Autodesk Inventor part; units mm, degrees
ref_plane "YZ Plane" through (0, 0, 0) normal (1, 0, 0) x (0, 1, 0)
ref_plane "XZ Plane" through (0, 0, 0) normal (0, 1, 0) x (-1, 0, 0)
ref_plane "XY Plane" through (0, 0, 0) normal (0, 0, 1) x (1, 0, 0)
sketch "Sketch1" plane through (0, 0, 0) normal (0, 1, 0) x (-1, 0, 0)
  line L0 (0, 0) -> (6, 0)
  line L1 (6, 0) -> (6, -3.7)
  line L2 (6, -3.7) -> (5, -3.7)
  line L3 (5, -3.7) -> (5, -8.7)
  line L4 (5, -8.7) -> (1, -8.7)
  line L5 (1, -8.7) -> (1, -3.7)
  line L6 (1, -3.7) -> (0, -3.7)
  line L7 (0, -3.7) -> (0, 0)
  dimension "d0" = 6
  dimension "d1" = 3.7
  dimension "d2" = 1
  dimension "d3" = 5
  dimension "d4" = 4
  dimension "d5" = 5
  dimension "d6" = 1
extrude "Extrusion1" add sketch "Sketch1" along normal blind 3
fillet "Fillet1" radius 1 2 edges at (-1, 1.5, -8.7) (-5, 1.5, -8.7)
properties part number "BBGW Case Button" material "Acrylic, Clear"
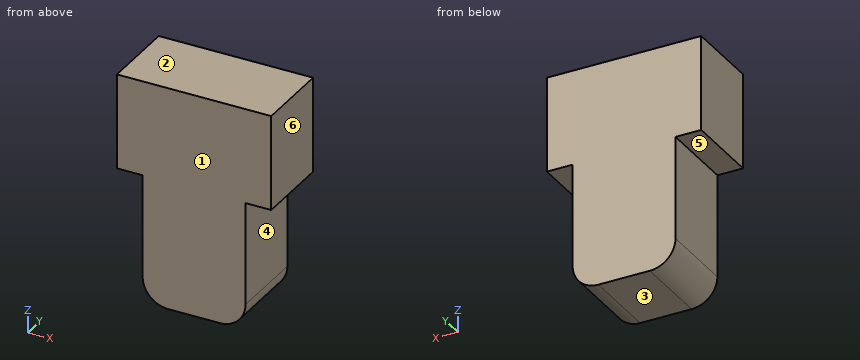
Here's how the part is built. I have some questions about the finished solid (model axes, mm). Face numbers are marked on the shaded views. A direction names the side the tool comes from. Coordinates: 2 decimals unless noted, no trailing zeros. Order: outer loops, then holes, each group sorted by start corner. A loop starts at its lowest first (then second) coordinate and runs counter-clockwise, first axis right, second up. Notation, with made-up numbers: M 23.25,67.5 L 64.25,67.5 A31 cw 64.25,104.5 Z; hole C 7,18.25 d3. An arc over 180 degrees is marked long. Answer as a JSON object with one key per item and string values. Group by question number.
(1) If we mould it in two halves opening along Z, with no side actions, what happens to the marked faces 1, 2 and 3? For each: released by +Z, released by -Z, zero draft, split by the parting line, or undercut.
(2) Which directions (+Z, -Z, +X, -X, +Y, -Y) give clear straight access to the entire face, cutting with the end or side of a thin tool? Please do the marked faces 4, 5 and 6.
(3) For pin 1 (0.5 mm diameter, centred on x = -0.5, y = 1.5, fed in from -Z); pin 2 (1.5 mm diameter, centred on x = -0.5, y = 2.5, fed in from -Z); pin 3 (1.5 mm diameter, centred on y = 1.5, z = -6.5, fed in from +X), each with a flat end and sliding along its axis, tell me the tip position at first contact or that it passes through.
(4) Suppose I cut it at A-A, the plane y = 2.6. Please give me the cut outline in (x, z), then the cut area to 3 significant figures.
(5) Suppose I cut it at B-B, the plane z = -7.25. Please give me the cut outline in (x, y), then the cut area to 3 significant figures.
(6) I need wall thicknesses on probe 1 along X at (y, z) = (2.1, -6.5); probe 2 along Z at (x, y) = (-5.25, 1.3); probe 3 along Z at (x, y) = (-1.1, 2.05). Which ranges of each line are inside material? Lowest first, please.
(7) Suppose I cut it at C-C, the plane x = -4.7. Please give me the cut outline in (y, z), then the cut area to 3 significant figures.
Values found:
{
 "1": {"face 1": "zero draft", "face 2": "released by +Z", "face 3": "released by -Z"},
 "2": {"face 4": "-Z, +X, +Y, -Y", "face 5": "-Z, -X, +Y, -Y", "face 6": "+Z, -Z, +X, +Y, -Y"},
 "3": {"pin 1": "stops at z = -3.7", "pin 2": "stops at z = -8.36", "pin 3": "stops at x = -1"},
 "4": {"outline": "M -6,-3.7 L -5,-3.7 L -5,-7.7 A1 ccw -4,-8.7 L -2,-8.7 A1 ccw -1,-7.7 L -1,-3.7 L 0,-3.7 L 0,0 L -6,0 Z", "area": "41.8 mm^2"},
 "5": {"outline": "M -5,0 L -1,0 L -1,3 L -5,3 Z", "area": "12.0 mm^2"},
 "6": {"probe 1": "x = -5 to -1", "probe 2": "z = -3.7 to 0", "probe 3": "z = -8.14 to 0"},
 "7": {"outline": "M 0,-8.41 L 3,-8.41 L 3,0 L 0,0 Z", "area": "25.2 mm^2"}
}
